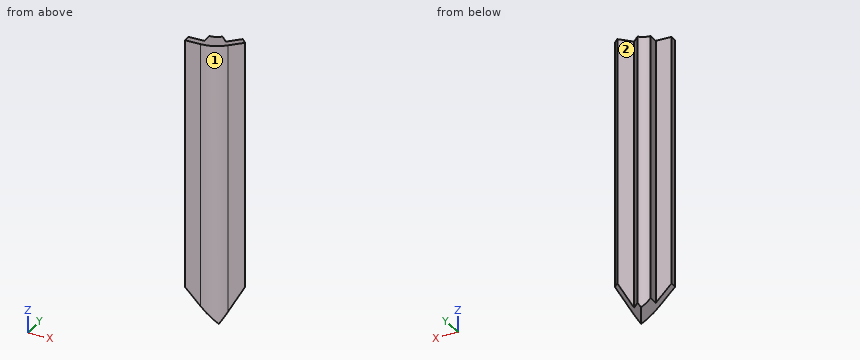
from build123d import *

# Parameters (mm, degrees)
SKETCH7_W               = 4.7625
SKETCH7_H               = 2.12122512
BOSS_EXTRUDE2_DEPTH     = 130.175
BOSS_EXTRUDE3_DEPTH     = 130.175
BOSS_EXTRUDE4_DEPTH     = 130.175
CUT_EXTRUDE1_DEPTH      = 1
CUT_EXTRUDE1_DEPTH_BACK = 118.807865064
SKETCH18_W              = 254
SKETCH18_H              = 254
CUT_EXTRUDE2_DEPTH      = 80.261506


with BuildPart() as part:
    # Sketch7 → Boss-Extrude2 (new body, symmetric)
    with BuildSketch(Plane.XY):
        with Locations((-4.92125, -2.560612608)):
            Rectangle(SKETCH7_W, SKETCH7_H)
    extrude(amount=BOSS_EXTRUDE2_DEPTH, both=True)



with BuildPart() as body_2:
    # Sketch8 → Boss-Extrude3 (new body, symmetric)
    with BuildSketch(Plane.XY):
        Polygon((2.85671143, 0.735391018), (6.224307475, 4.102987064), (7.724240142, 2.603054397), (4.356644097, -0.764541648), align=None)
    extrude(amount=BOSS_EXTRUDE3_DEPTH, both=True)


with BuildPart() as part_1:
    add(part.part)

    add(body_2.part)  # Boss-Extrude4 merges body 2
    # Sketch11 → Boss-Extrude4 (add, symmetric)
    with BuildSketch(Plane.XY):
        with BuildLine():
            Line((-2.54, -1.500000048), (-7.3025, -1.500000048))
            Line((-7.3025, -1.500000048), (-7.3025, -3.621225168))
            Line((-7.3025, -3.621225168), (-2.54, -3.621225168))
            ThreePointArc((-2.54, -3.621225168), (1.192436889, -2.87879731), (4.356644097, -0.764541648))
            Line((4.356644097, -0.764541648), (7.724240142, 2.603054397))
            Line((7.724240142, 2.603054397), (6.224307475, 4.102987064))
            Line((6.224307475, 4.102987064), (2.85671143, 0.735391018))
            Line((2.85671143, 0.735391018), (0.735391018, 2.85671143))
            ThreePointArc((0.735391018, 2.85671143), (-0.767371154, 1.852597848), (-2.54, 1.500000048))
            Line((-2.54, 1.500000048), (-2.54, -1.500000048))
        make_face()
    extrude(amount=BOSS_EXTRUDE4_DEPTH, both=True)

    # Sketch17 → Cut-Extrude1 (cut, two sides)
    with BuildSketch(Plane(origin=(47.098102576, -113.704878, 0), x_dir=(-1, 0, 0), z_dir=(0, -1, 0))) as cut_extrude1_sk:
        Polygon((-898.025612107, 898.025612107), (898.025612107, -898.025612107), (2694.076836321, 898.025612107), (898.025612107, 2694.076836321), align=None)
    extrude(amount=CUT_EXTRUDE1_DEPTH, mode=Mode.SUBTRACT)
    extrude(cut_extrude1_sk.sketch, amount=-CUT_EXTRUDE1_DEPTH_BACK, mode=Mode.SUBTRACT)

    # Sketch18 → Cut-Extrude2 (cut)
    with BuildSketch(Plane(origin=(47.098102576, 47.098102576, 0), x_dir=(0.816496581, -0.40824829, 0.40824829), z_dir=(0.577350269, 0.577350269, -0.577350269))):
        Rectangle(SKETCH18_W, SKETCH18_H)
    extrude(amount=-CUT_EXTRUDE2_DEPTH, mode=Mode.SUBTRACT)


solid = part_1.part
Build history of the part. All positions in model axes, mm. Face numbers are marked on the shaded views. Coordinates: 2 decimals unless noted, no trailing zeros. Order: outer loops, then holes, each group sorted by start corner. A loop starts at its lowest first (then second) coordinate and runs counter-clockwise, first axis right, second up. Notation, with made-up numbers: (89, 80) - (143, 80) arc R12 ccw to (143, 84) - close; hole circle Ø3 at (22.5, 57.5). An arc over 180 degrees is marked (long way). Write item = value, one per line. Start each with the question number.
1) Two-plate mould, pull along X, no slides. Class the marked faces 1 and 2: pulls with the +X half, pulls with the -X half, needs draft (parallel to the pull), parting line crosses it, or undercut.
2) Saw through at B-B on x = -1.5. Write the cut outline in (y, z) (3 decimals).
3) Wall check: line 1 along X through (y, z) = (1.25, 61); line 2 along Y through (x, z) = (-2.25, 114); line 3 along X through (y, z) = (1, 108). Give the ranges that are in metal, low to high. Write a range as from..to.
4) Flat gauge pins, fed straight in: pin 1 Ø1.5 at (y, z) = (0, 54.5) entering from +X; pin 2 Ø2 at (y, z) = (1, 112.5) entering from -X; pin 3 Ø4 at (x, z) = (-6, 108) entering from +Y. Where does each tip first touch, or does it go through?
5) Saw through at A-A on z = 86. Write the cut outline in (x, y).
From the geometry:
q1.face_1 = pulls with the +X half
q1.face_2 = undercut
q2.outline = (-3.566, 48.598) - (1.618, 48.598) - (1.618, 130.175) - (-3.566, 130.175) - close
q3.line_1 = -2.54..2.34, 3.37..6.37
q3.line_2 = -3.62..1.51
q3.line_3 = -2.54..2.59, 3.12..6.12
q4.pin_1 = 5.87
q4.pin_2 = -2.54
q4.pin_3 = -1.5
q5.outline = (-7.3, -3.62) - (-2.54, -3.62) arc R9.75 ccw to (4.36, -0.76) - (7.72, 2.6) - (6.22, 4.1) - (2.86, 0.74) - (0.74, 2.86) arc R4.63 cw to (-2.54, 1.5) - (-2.54, -1.5) - (-7.3, -1.5) - close
